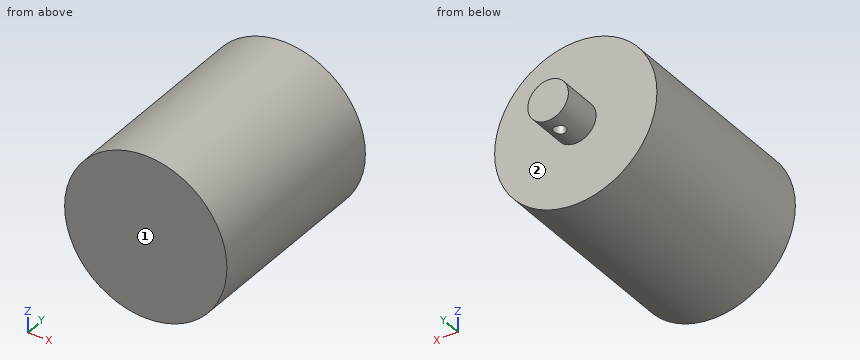
from build123d import *

# Parameters (mm, degrees)
SKETCH1_R           = 20
BOSS_EXTRUDE1_DEPTH = 50
SKETCH2_R           = 5
BOSS_EXTRUDE2_DEPTH = 10
SKETCH3_R           = 1.5
CUT_EXTRUDE1_DEPTH  = 16


with BuildPart() as part:
    # Sketch1 → Boss-Extrude1 (new body)
    with BuildSketch(Plane(origin=(0, 0, 0), x_dir=(1, 0, 0), z_dir=(0, 1, 0))):
        with Locations(Location((0, 0, 0), (0, 0, 270))):
            Circle(SKETCH1_R)
    extrude(amount=BOSS_EXTRUDE1_DEPTH)

    # Sketch2 → Boss-Extrude2 (add)
    with BuildSketch(Plane(origin=(0, 50, 0), x_dir=(1, 0, 0), z_dir=(0, 1, 0))):
        with Locations(Location((0, 0, 0), (0, 0, 270))):
            Circle(SKETCH2_R)
    extrude(amount=BOSS_EXTRUDE2_DEPTH)

    # Sketch3 → Cut-Extrude1 (cut)
    with BuildSketch(Plane.XY):
        with Locations((0, 55.836490144)):
            Circle(SKETCH3_R)
    extrude(amount=-CUT_EXTRUDE1_DEPTH, mode=Mode.SUBTRACT)


solid = part.part
Model file for the job. Use its own axes, mm. Face numbers are marked on the shaded views. A direction names the side the tool comes from. Coordinates: 2 decimals unless noted, no trailing zeros. Loops run counter-clockwise (first coordinate to the right, second up) from the corner with the lowest first, then second, coordinate; pieces in that order, holes last. Notation, with made-up numbers: (62, -6) -> (83, -6) arc R25 cw to (83, 30) -> close; hole circle Ø3 at (-21.75, 64). An arc over 180 degrees is marked (long way). Use one line per item in the form item = value. Start each with the question number.
(1) Probe probe 1 along Y at (x, z) = (0, -3); probe 2 along Y at (x, z) = (8, -15.5); probe 3 along X at (y, z) = (44, 14.5). List the from-to ranges inside material, lowest first. Write a range as from..to.
(2) Cut at D-D on x = 16. Give the cut face in (y, z).
(3) Tool access for the marked faces 1 and 2: list every direction of +Z, -Z, +X, -X, +Y, -Y with a clear straight run to the whole face (end or side of a thin tool).
(4) Cut at A-A on x = 0. Give the cut face in (y, z).
(5) Cut at C-C on z = 9. Give the cut face in (x, y).
(6) Cut at B-B on y = 21.5. Give the cut face in (x, z), and give its area (3 significant figures).
(7) Flat gauge pins, fed straight in: pin 1 (10 mm diameter, centred on y = 11.5, z = -10.5, fed in from -X); pin 2 (10 mm diameter, centred on y = 53, z = 1, fed in from -X); pin 3 (10 mm diameter, centred on x = -13.5, y = 15.5, fed in from +Z). Where does each tip first touch, or does it go through?
Values:
q1.probe_1 = 0..54.34, 57.34..60
q1.probe_2 = 0..50
q1.probe_3 = -13.77..13.77
q2.outline = (0, -12) -> (50, -12) -> (50, 12) -> (0, 12) -> close
q3.face_1 = +Z, -Z, +X, -X, -Y
q3.face_2 = +Y
q4.outline = (0, -20) -> (50, -20) -> (50, -5) -> (54.34, -5) -> (54.34, 0) -> (57.34, 0) -> (57.34, -5) -> (60, -5) -> (60, 5) -> (50, 5) -> (50, 20) -> (0, 20) -> close
q5.outline = (-17.86, 0) -> (17.86, 0) -> (17.86, 50) -> (-17.86, 50) -> close
q6.outline = circle Ø40 at (0, 0)
q6.area = 1,260 mm2
q7.pin_1 = -19.23
q7.pin_2 = -20
q7.pin_3 = 18.1
